Could you check a few things on this drawing? It's one solid part, dimensions in mm from its lowest x, y, z. A direction names the side the tool comes from. Give positions to 0.01 mm unless a question says otherwise; leave off trailing zeros. Write each loop counter-clockwise with the first axis right and the second up, starting at its lowest first coordinate (ties: lowest second). Pieces come first, ordered by that corner, then holes.
1. On a 3-axis mill with a long thin cutter (end or side, diameter ignored), from which of +Z, -Z, +X, -X, +Y, -Y can I reach the whole of each face in a straight line? I mean the marked faces 1, 2, 3, 4 and 5. Say none if no direction works.
2. I'm going to push flat-ended pins straight in: pin 1 (3.5 mm diameter, centred on x = 3.5, y = 1.5, fed in from -Z); pin 2 (3 mm diameter, centred on y = 3.5, z = 9.5, fed in from +X); pin 3 (0.8 mm diameter, centred on x = 5, y = 6, fed in from -Z); pin 4 (2 mm diameter, centred on y = 1, z = 14.5, fed in from +X). Where does each tip first touch, or does it pass through?
3. Suppose I cut it at C-C (z = 19.5). Please give me the cut outline in (x, y).
4. Thinking about a two-plate mould opening in Z: for the marked faces 6, 7 and 8, which applies, pulls with the +Z half, pulls with the -Z half, needs draft (parallel to the pull), parting line crosses it, or undercut?
5. Suppose I cut it at B-B (y = 4.5). Please give me the cut outline in (x, z), and give its area (3 significant figures).
6. If I drill on probe 1 along Z at (x, y) = (4.25, 1); probe 2 along Y at (x, z) = (3.5, 9.5); probe 3 along X at (y, z) = (5, 11.5), over which ranges is the centre line in solid material (lowest first)?
7. Suppose I cut it at A-A (x = 5.75). Please give me the cut outline in (y, z).
8. Suppose I cut it at D-D (x = 4). Please give me the cut outline in (y, z).
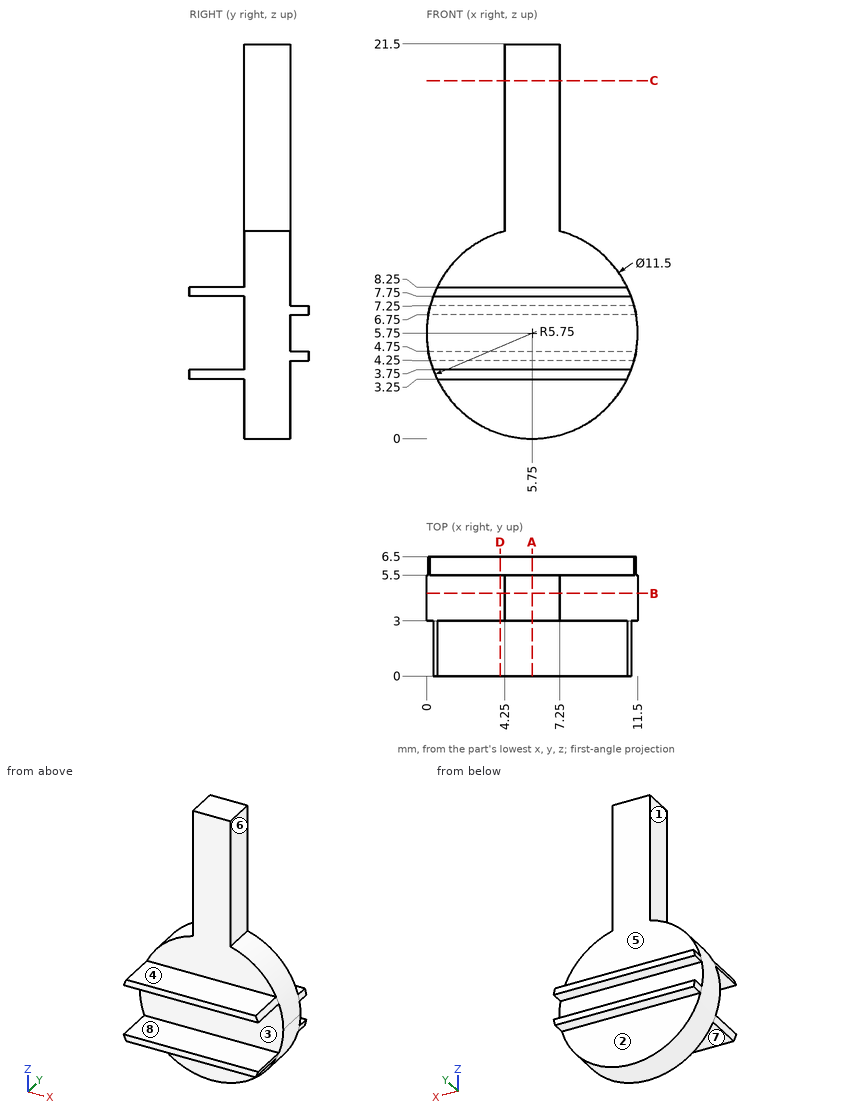
Checks:
1. face 1: +Z, -X, +Y, -Y
1. face 2: -Z, +X, -X, +Y
1. face 3: +X, -X, -Y
1. face 4: +Z, +X, -X, -Y
1. face 5: +Z, +X, -X, +Y
2. pin 1: stops at z = 0.16
2. pin 2: stops at x = 11.04
2. pin 3: stops at z = 4.25
2. pin 4: passes through
3. outline: (4.25, 3) - (7.25, 3) - (7.25, 5.5) - (4.25, 5.5) - close
4. face 6: needs draft
4. face 7: pulls with the -Z half
4. face 8: undercut
5. outline: (4.25, 11.3) arc R5.75 ccw (long way) to (7.25, 11.3) - (7.25, 21.5) - (4.25, 21.5) - close
5. area: 134 mm2
6. probe 1: z = 3.25 to 3.75, 7.75 to 8.25
6. probe 2: y = 3 to 5.5
6. probe 3: x = 4.25 to 7.25
7. outline: (0, 3.25) - (3, 3.25) - (3, 0) - (5.5, 0) - (5.5, 4.25) - (6.5, 4.25) - (6.5, 4.75) - (5.5, 4.75) - (5.5, 6.75) - (6.5, 6.75) - (6.5, 7.25) - (5.5, 7.25) - (5.5, 21.5) - (3, 21.5) - (3, 8.25) - (0, 8.25) - (0, 7.75) - (3, 7.75) - (3, 3.75) - (0, 3.75) - close
8. outline: (0, 3.25) - (3, 3.25) - (3, 0.27) - (5.5, 0.27) - (5.5, 4.25) - (6.5, 4.25) - (6.5, 4.75) - (5.5, 4.75) - (5.5, 6.75) - (6.5, 6.75) - (6.5, 7.25) - (5.5, 7.25) - (5.5, 11.23) - (3, 11.23) - (3, 8.25) - (0, 8.25) - (0, 7.75) - (3, 7.75) - (3, 3.75) - (0, 3.75) - close
